Source: CAD feature listing. Evaluate the final solid. Frame: model axes, mm. A direction names the side the tool comes from. Coordinates: 2 decimals unless noted, no trailing zeros. Write each loop counter-clockwise with the first axis right and the second up, starting at its lowest first coordinate (ties: lowest second). Pieces come first, ordered by that corner, then holes. Notation, with made-up numbers: M -34.5,26.5 L -24.5,26.5 A20 cw -24.5,49.5 Z; hole C 63.25,-32 d4. An arc over 180 degrees is marked long. Write item = value, one per line. Start each with the question number.
1. Line query: line 1 along X through (y, z) = (-5.5, 41); line 2 along X through (y, z) = (3.75, -69.5); line 3 along X through (y, z) = (0, -17.5). Output: solid intervals per line, ascending.
2. Pull-direction query (X, two-part tool) for faces 5 (the face through (12.7, 8, 1)), 6 (the face through (7.04, -5.48, 1.07)), 7 (the face through (0.782, 2.483, 1.067)), 8 (the face through (-8, -12.7, 1)); classes: pulls with the +X half, pulls with the -X half, needs draft (parallel to the pull), parting line crosses it, or undercut.
3. Pin query (flat end, axial travel): pin 1 Ø3.5 at (x, z) = (0, -2.5) entering from -Y; pin 2 Ø1 at (x, z) = (-1, 11) entering from +Y; pin 3 Ø3.5 at (y, z) = (-0.5, -23.5) entering from -X. Return the tip coordinate at first contact, or that it passes through.
4. Access query for faces 1 (the face through (-4.517, 0, 1)), 2 (the face through (-5.48, -7.04, 1.07)), 3 (the face through (0, -4.517, 1)), 4 (the face through (0, 4.517, 1)). Directions: +Z, -Z, +X, -X, +Y, -Y. A direction counts if a zero-diameter tool reaches every point of the face in a straight line with its end or side. Return the directions, or none.
5. Section query A-A (y = 0). Output: boundary loops of the cut face in (x, z), then the cut area to 3 significant figures.
```python
from build123d import *

# Parameters (mm, degrees)
SKETCH11_R              = 2.6035
FRACTIONAL_1010_1_DEPTH = 152.4


with BuildPart() as part:
    # Sketch11 → Fractional 1010(1) (new body)
    with BuildSketch(Plane.YX.offset(-76.2)):
        with BuildLine():
            Line((10.5918, 12.7), (10.5664, 12.7))
            ThreePointArc((10.5664, 12.7), (10.0584, 12.192), (9.5504, 12.7))
            Line((9.5504, 12.7), (6.3246, 12.7))
            ThreePointArc((6.3246, 12.7), (5.8166, 12.192), (5.3086, 12.7))
            Line((5.3086, 12.7), (4.3561, 12.7))
            ThreePointArc((4.3561, 12.7), (3.2512, 11.5951), (4.3561, 10.4902))
            Line((4.3561, 10.4902), (6.370083786, 10.4902))
            ThreePointArc((6.370083786, 10.4902), (7.348856743, 9.836204819), (7.119204175, 8.681663397))
            Line((7.119204175, 8.681663397), (3.88464389, 5.447103113))
            ThreePointArc((3.88464389, 5.447103113), (2.854599758, 4.758849627), (1.63957986, 4.517167143))
            Line((1.63957986, 4.517167143), (-1.63957986, 4.517167143))
            ThreePointArc((-1.63957986, 4.517167143), (-2.854599758, 4.758849627), (-3.88464389, 5.447103113))
            Line((-3.88464389, 5.447103113), (-7.119204175, 8.681663397))
            ThreePointArc((-7.119204175, 8.681663397), (-7.348856743, 9.836204819), (-6.370083786, 10.4902))
            Line((-6.370083786, 10.4902), (-4.3561, 10.4902))
            ThreePointArc((-4.3561, 10.4902), (-3.2512, 11.5951), (-4.3561, 12.7))
            Line((-4.3561, 12.7), (-5.3086, 12.7))
            ThreePointArc((-5.3086, 12.7), (-5.8166, 12.192), (-6.3246, 12.7))
            Line((-6.3246, 12.7), (-9.5504, 12.7))
            ThreePointArc((-9.5504, 12.7), (-10.0584, 12.192), (-10.5664, 12.7))
            Line((-10.5664, 12.7), (-10.5918, 12.7))
            ThreePointArc((-10.5918, 12.7), (-12.082522516, 12.082522516), (-12.7, 10.5918))
            Line((-12.7, 10.5918), (-12.7, 10.5664))
            ThreePointArc((-12.7, 10.5664), (-12.192, 10.0584), (-12.7, 9.5504))
            Line((-12.7, 9.5504), (-12.7, 6.3246))
            ThreePointArc((-12.7, 6.3246), (-12.192, 5.8166), (-12.7, 5.3086))
            Line((-12.7, 5.3086), (-12.7, 4.3561))
            ThreePointArc((-12.7, 4.3561), (-11.5951, 3.2512), (-10.4902, 4.3561))
            Line((-10.4902, 4.3561), (-10.4902, 6.370083786))
            ThreePointArc((-10.4902, 6.370083786), (-9.836204819, 7.348856743), (-8.681663397, 7.119204175))
            Line((-8.681663397, 7.119204175), (-5.447103113, 3.88464389))
            ThreePointArc((-5.447103113, 3.88464389), (-4.758849627, 2.854599758), (-4.517167143, 1.63957986))
            Line((-4.517167143, 1.63957986), (-4.517167143, -1.63957986))
            ThreePointArc((-4.517167143, -1.63957986), (-4.758849627, -2.854599758), (-5.447103113, -3.88464389))
            Line((-5.447103113, -3.88464389), (-8.681663397, -7.119204175))
            ThreePointArc((-8.681663397, -7.119204175), (-9.836204819, -7.348856743), (-10.4902, -6.370083786))
            Line((-10.4902, -6.370083786), (-10.4902, -4.3561))
            ThreePointArc((-10.4902, -4.3561), (-11.5951, -3.2512), (-12.7, -4.3561))
            Line((-12.7, -4.3561), (-12.7, -5.3086))
            ThreePointArc((-12.7, -5.3086), (-12.192, -5.8166), (-12.7, -6.3246))
            Line((-12.7, -6.3246), (-12.7, -9.5504))
            ThreePointArc((-12.7, -9.5504), (-12.192, -10.0584), (-12.7, -10.5664))
            Line((-12.7, -10.5664), (-12.7, -10.5918))
            ThreePointArc((-12.7, -10.5918), (-12.082522516, -12.082522516), (-10.5918, -12.7))
            Line((-10.5918, -12.7), (-10.5664, -12.7))
            ThreePointArc((-10.5664, -12.7), (-10.0584, -12.192), (-9.5504, -12.7))
            Line((-9.5504, -12.7), (-6.3246, -12.7))
            ThreePointArc((-6.3246, -12.7), (-5.8166, -12.192), (-5.3086, -12.7))
            Line((-5.3086, -12.7), (-4.3561, -12.7))
            ThreePointArc((-4.3561, -12.7), (-3.2512, -11.5951), (-4.3561, -10.4902))
            Line((-4.3561, -10.4902), (-6.370083786, -10.4902))
            ThreePointArc((-6.370083786, -10.4902), (-7.348856743, -9.836204819), (-7.119204175, -8.681663397))
            Line((-7.119204175, -8.681663397), (-3.88464389, -5.447103113))
            ThreePointArc((-3.88464389, -5.447103113), (-2.854599758, -4.758849627), (-1.63957986, -4.517167143))
            Line((-1.63957986, -4.517167143), (1.63957986, -4.517167143))
            ThreePointArc((1.63957986, -4.517167143), (2.854599758, -4.758849627), (3.88464389, -5.447103113))
            Line((3.88464389, -5.447103113), (7.119204175, -8.681663397))
            ThreePointArc((7.119204175, -8.681663397), (7.348856743, -9.836204819), (6.370083786, -10.4902))
            Line((6.370083786, -10.4902), (4.3561, -10.4902))
            ThreePointArc((4.3561, -10.4902), (3.2512, -11.5951), (4.3561, -12.7))
            Line((4.3561, -12.7), (5.3086, -12.7))
            ThreePointArc((5.3086, -12.7), (5.8166, -12.192), (6.3246, -12.7))
            Line((6.3246, -12.7), (9.5504, -12.7))
            ThreePointArc((9.5504, -12.7), (10.0584, -12.192), (10.5664, -12.7))
            Line((10.5664, -12.7), (10.5918, -12.7))
            ThreePointArc((10.5918, -12.7), (12.082522516, -12.082522516), (12.7, -10.5918))
            Line((12.7, -10.5918), (12.7, -10.5664))
            ThreePointArc((12.7, -10.5664), (12.192, -10.0584), (12.7, -9.5504))
            Line((12.7, -9.5504), (12.7, -6.3246))
            ThreePointArc((12.7, -6.3246), (12.192, -5.8166), (12.7, -5.3086))
            Line((12.7, -5.3086), (12.7, -4.3561))
            ThreePointArc((12.7, -4.3561), (11.5951, -3.2512), (10.4902, -4.3561))
            Line((10.4902, -4.3561), (10.4902, -6.370083786))
            ThreePointArc((10.4902, -6.370083786), (9.836204819, -7.348856743), (8.681663397, -7.119204175))
            Line((8.681663397, -7.119204175), (5.447103113, -3.88464389))
            ThreePointArc((5.447103113, -3.88464389), (4.758849627, -2.854599758), (4.517167143, -1.63957986))
            Line((4.517167143, -1.63957986), (4.517167143, 1.63957986))
            ThreePointArc((4.517167143, 1.63957986), (4.758849627, 2.854599758), (5.447103113, 3.88464389))
            Line((5.447103113, 3.88464389), (8.681663397, 7.119204175))
            ThreePointArc((8.681663397, 7.119204175), (9.836204819, 7.348856743), (10.4902, 6.370083786))
            Line((10.4902, 6.370083786), (10.4902, 4.3561))
            ThreePointArc((10.4902, 4.3561), (11.5951, 3.2512), (12.7, 4.3561))
            Line((12.7, 4.3561), (12.7, 5.3086))
            ThreePointArc((12.7, 5.3086), (12.192, 5.8166), (12.7, 6.3246))
            Line((12.7, 6.3246), (12.7, 9.5504))
            ThreePointArc((12.7, 9.5504), (12.192, 10.0584), (12.7, 10.5664))
            Line((12.7, 10.5664), (12.7, 10.5918))
            ThreePointArc((12.7, 10.5918), (12.082522516, 12.082522516), (10.5918, 12.7))
        make_face()
        Circle(SKETCH11_R, mode=Mode.SUBTRACT)
    extrude(amount=FRACTIONAL_1010_1_DEPTH)


solid = part.part
```
Results are:
q1.line_1 = -12.3 to -10.49, -7.06 to -3.94, 3.94 to 7.06, 10.49 to 12.3
q1.line_2 = -12.52 to -10.67, -5.32 to 5.32, 10.67 to 12.52
q1.line_3 = -4.52 to -2.6, 2.6 to 4.52
q2.face_5 = pulls with the +X half
q2.face_6 = undercut
q2.face_7 = undercut
q2.face_8 = needs draft
q3.pin_1 = -4.52
q3.pin_2 = 4.52
q3.pin_3 = -4.58
q4.face_1 = +Z, -Z, -X
q4.face_2 = +Z, -Z
q4.face_3 = +Z, -Z, -Y
q4.face_4 = +Z, -Z, +Y
q5.outline = M -4.52,-76.2 L -2.6,-76.2 L -2.6,76.2 L -4.52,76.2 Z; M 2.6,-76.2 L 4.52,-76.2 L 4.52,76.2 L 2.6,76.2 Z
q5.area = 583 mm^2
